The figure shows three views and two pictorial views of one solid part (mm, origin at its lowest corner). Answer the questions. A direction names the side the tool comes from. Round coordinates to 2 decimals unless told otherwise and drop trailing zeros. Order: outer loops, then holes, each group sorted by start corner. A loop starts at its lowest first (then second) coordinate and runs counter-clockwise, first axis right, second up. Notation, with made-up numbers: (23.5, 21.25) -> (71.5, 21.25) arc R22 ccw to (71.5, 35.25) -> close; hole circle Ø3 at (63.25, 12). An arc over 180 degrees is marked (long way). Return JSON: item names as keys, results as strings. Group by question number.
(1) The part is cut by section B-B (x = 3.75). Determine the outline of the cut face in (y, z).
(2) The part is cut by section C-C (z = 9). Determine the outline of the cut face in (x, y), plus the area to 3 significant figures.
(3) Each of these flat-tipped pins is pushed along its axis until it touches: pin 1 (1.2 mm diameter, centred on x = 4.5, z = 7.5, fed in from -Y); pin 2 (2 mm diameter, centred on x = 3, z = 5.5, fed in from +Y); pin 3 (6 mm diameter, centred on y = 10.5, z = 9, fed in from -X). Where does it stop, or does it pass through?
(4) Which of the six approach directions +Z, -Z, +X, -X, +Y, -Y give full straight-line access (tool end or side, diameter ignored) to the marked faces 1, 2, 3 and 4?
(5) The part is cut by section A-A (y = 25). Determine the outline of the cut face in (x, z), plus the area to 3 significant figures.
(6) Consider line 1 (X direction, y = 43, z = 7); line 2 (Z direction, x = 1.75, y = 38). Determine where each line is inside the solid, lowest interval first. Write a range as [from, to].
(7) The part is cut by section D-D (x = 9.25). Determine the outline of the cut face in (y, z).
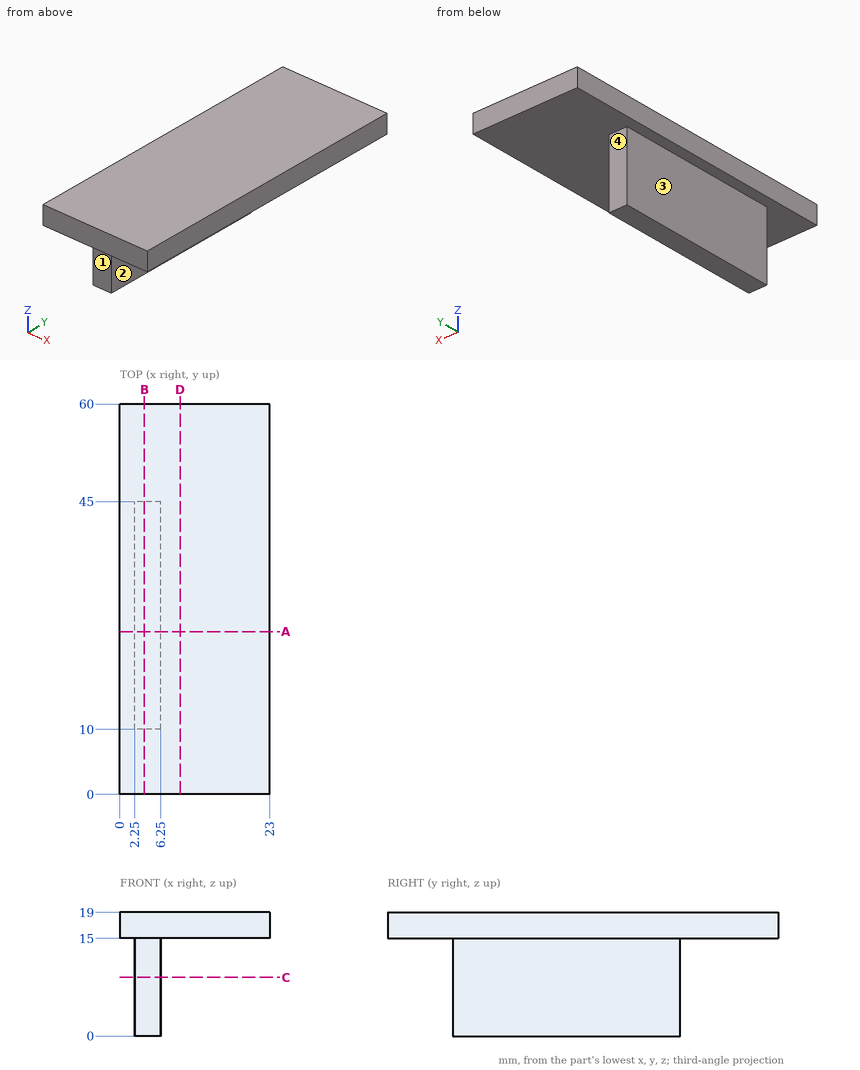
Answer below:
{
 "1": {"outline": "(0, 15) -> (10, 15) -> (10, 0) -> (45, 0) -> (45, 15) -> (60, 15) -> (60, 19) -> (0, 19) -> close"},
 "2": {"outline": "(2.25, 10) -> (6.25, 10) -> (6.25, 45) -> (2.25, 45) -> close", "area": "140 mm²"},
 "3": {"pin 1": "stops at y = 10", "pin 2": "stops at y = 45", "pin 3": "stops at x = 2.25"},
 "4": {"face 1": "-Z, +X, -X, -Y", "face 2": "-Z, +X, +Y, -Y", "face 3": "-Z, -X, +Y, -Y", "face 4": "-Z, +X, -X, +Y"},
 "5": {"outline": "(0, 15) -> (2.25, 15) -> (2.25, 0) -> (6.25, 0) -> (6.25, 15) -> (23, 15) -> (23, 19) -> (0, 19) -> close", "area": "152 mm²"},
 "6": {"line 1": "x = [2.25, 6.25]", "line 2": "z = [15, 19]"},
 "7": {"outline": "(0, 15) -> (60, 15) -> (60, 19) -> (0, 19) -> close"}
}
